Part print with two shaded views. Sizes in mm from the minimum x, y, z corner. A direction names the side the tool comes from. Give positions to 0.01 mm unless a question says otherwise; leave off trailing zeros. Order: outer loops, then holes, each group sorted by start corner. A loop starts at its lowest first (then second) coordinate and runs counter-clockwise, first axis right, second up. Notation, with made-up numbers: M 12,38 L 34,38 A23 cw 34,68 Z; hole C 80.5,-24.75 d2. An arc over 180 degrees is marked long. Return JSON: item names as keys, results as strings.
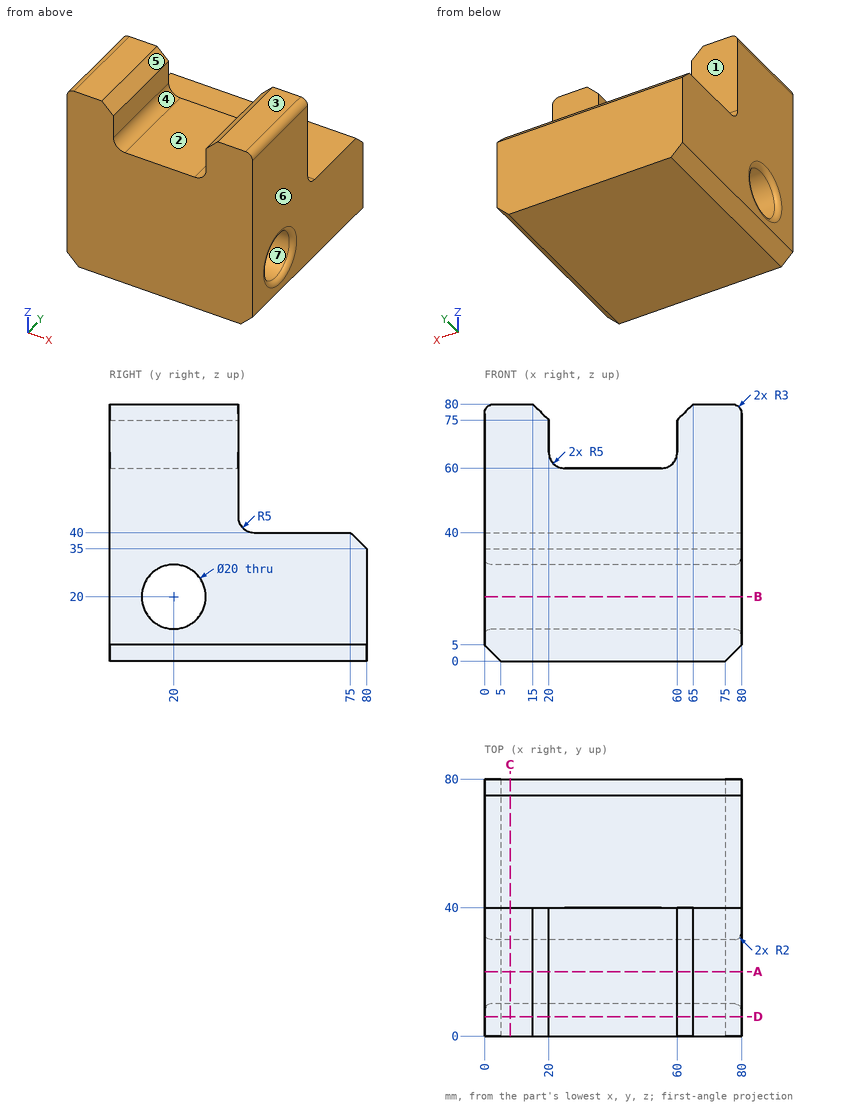
Q1. Band-saw the part on B-B (z = 20). Give the cut face in (x, y).
Established:
{"outline": "M 0,0 L 80,0 L 80,8 A2 ccw 78,10 L 2,10 A2 ccw 0,8 Z; M 0,32 A2 ccw 2,30 L 78,30 A2 ccw 80,32 L 80,80 L 0,80 Z"}
Q2. Two-plate mould, pull along X, no slides. Class the marked faces 4, 5, 6 and 7: +X half, -X half, draft (parallel to the pull), parting line (faces both ways), or undercut.
Established:
{"face 4": "undercut", "face 5": "undercut", "face 6": "+X half", "face 7": "draft"}
Q3. Probe line 1 along Y through (x, z) = (38, 20); line 2 along Z through (x, y) = (37, 33); line 3 along Z through (x, y) = (32, 23). List the from-to ranges inside material, lowest first.
Established:
{"line 1": "y = 0 to 10, 30 to 80", "line 2": "z = 0 to 60", "line 3": "z = 0 to 10.46, 29.54 to 60"}
Q4. Pin check, flat tips, straight feed: pin 1 (15 mm diameter, centred on x = 44.5, y = 24, fed in from +Z); pin 2 (24 mm diameter, centred on x = 27, y = 61, fed in from +Z). Stop position of each tip, or through.
Established:
{"pin 1": "stops at z = 60", "pin 2": "stops at z = 40"}
Q5. 3-axis set-ups, long thin cutter, end or side, ignore diameter. For the marked faces 1, 2 and 3: which of +Z, -Z, +X, -X, +Y, -Y reach the whole face in a straight line?
Established:
{"face 1": "+Z, +X, -X, +Y", "face 2": "+Z, +Y, -Y", "face 3": "+Z, +X, -X, +Y, -Y"}
Q6. Band-saw the part on D-D (y = 6). Give the cut face in (x, z).
Established:
{"outline": "M 0,5 L 5,0 L 75,0 L 80,5 L 80,77 A3 ccw 77,80 L 65,80 L 60,75 L 60,65 A5 cw 55,60 L 25,60 A5 cw 20,65 L 20,75 L 15,80 L 3,80 A3 ccw 0,77 Z"}
Q7. Band-saw the part on C-C (x = 8). Give the cut face in (y, z).
Established:
{"outline": "M 0,0 L 80,0 L 80,35 L 75,40 L 45,40 A5 cw 40,45 L 40,80 L 0,80 Z; hole C 20,20 d20"}
Q8. Band-saw the part on A-A (y = 20). Give the cut face in (x, z), then the cut area to 3 significant figures.
Established:
{"outline": "M 0,5 L 5,0 L 75,0 L 80,5 L 80,8 A2 ccw 78,10 L 2,10 A2 ccw 0,8 Z; M 0,32 A2 ccw 2,30 L 78,30 A2 ccw 80,32 L 80,77 A3 ccw 77,80 L 65,80 L 60,75 L 60,65 A5 cw 55,60 L 25,60 A5 cw 20,65 L 20,75 L 15,80 L 3,80 A3 ccw 0,77 Z", "area": "3,950 mm²"}
